Geometry check sheet. Reference: drawing and pictorial views, mm from the part's lowest x, y, z. A direction names the side the tool comes from. Round coordinates to 2 decimals unless told otherwise and drop trailing zeros. Order: outer loops, then holes, each group sorted by start corner. A loop starts at its lowest first (then second) coordinate and runs counter-clockwise, first axis right, second up. Notation, with made-up numbers: (8.5, 60.25) -> (22.5, 60.25) arc R31 cw to (22.5, 91.25) -> close; hole circle Ø5 at (-31.75, 65). An arc over 180 degrees is marked (long way). Put each result on its own line as item: value.
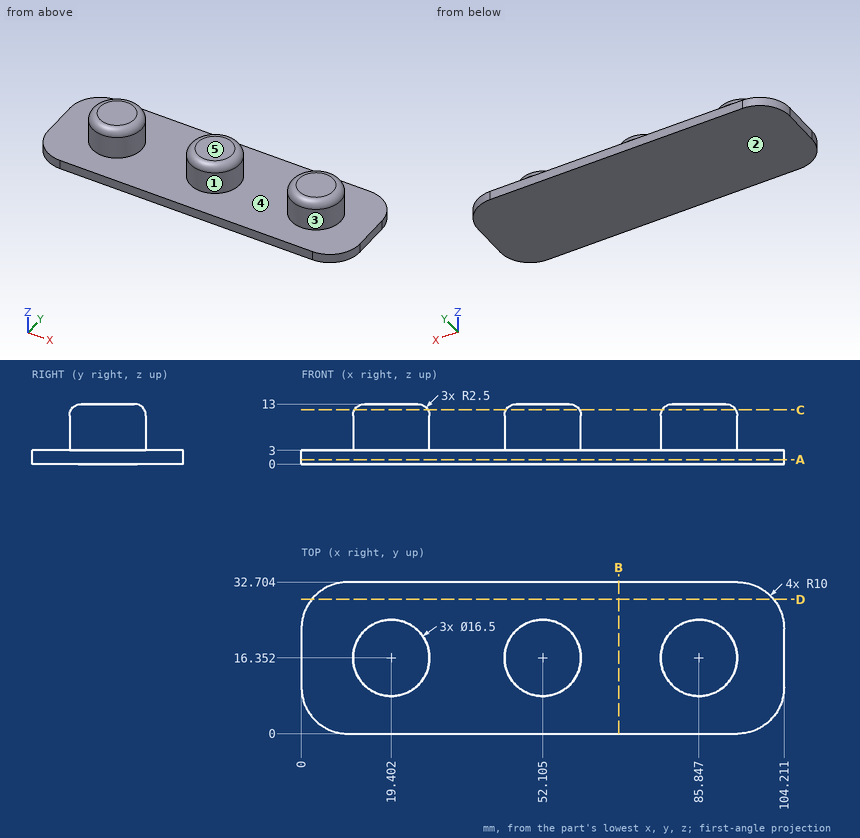
Item 1: Tool access check on the marked faces 1 and 2. Record the directions out of +Z, -Z, +X, -X, +Y, -Y that give a thin tool (end or side, any length) a straight path to the whole face; none if there is none.
Geometry check:
face 1: +Z
face 2: -Z, +X, -X, +Y, -Y
Item 2: Sectioned sample at B-B, the plane x = 68.5. Record the boundary of the cut face in (y, z).
Geometry check:
outline: (0, 0) -> (32.7, 0) -> (32.7, 3) -> (0, 3) -> close
Item 3: Material ranges on line 1 along X through (y, z) = (11.5, 8) (1 decimal); line 2 along X through (y, z) = (12, 7.25) (1 decimal); line 3 along Z through (x, y) = (92, 26), recorded low to high.
Geometry check:
line 1: 12.7 to 26.1, 45.4 to 58.8, 79.2 to 92.5
line 2: 12.4 to 26.4, 45.1 to 59.1, 78.8 to 92.9
line 3: 0 to 3
Item 4: Sectioned sample at D-D, the plane y = 29. Record the boundary of the cut face in (x, z), then the cut area to 3 significant figures.
Geometry check:
outline: (2.23, 0) -> (101.98, 0) -> (101.98, 3) -> (2.23, 3) -> close
area: 299 mm2
Item 5: Release check for a two-part mould opening along X. For the marked faces 3, 4 and 5 record: pulls with the +X half, pulls with the -X half, needs draft (parallel to the pull), parting line crosses it, or undercut.
Geometry check:
face 3: undercut
face 4: undercut
face 5: needs draft
Item 6: Sectioned sample at A-A, the plane z = 1. Record the boundary of the cut face in (x, y), then the cut area to 3 significant figures.
Geometry check:
outline: (0, 10) arc R10 ccw to (10, 0) -> (94.21, 0) arc R10 ccw to (104.21, 10) -> (104.21, 22.7) arc R10 ccw to (94.21, 32.7) -> (10, 32.7) arc R10 ccw to (0, 22.7) -> close
area: 3,320 mm2
Item 7: Depth check by flat-ended pin: pin 1 Ø2 at (x, y) = (94, 19) entering from +Z; pin 2 Ø2 at (x, z) = (82.5, 5.5) entering from +Y; pin 3 Ø6 at (y, z) = (7.5, 9) entering from -X (1 decimal). Enter the tip coordinate at first touch or a pass-through.
Geometry check:
pin 1: z = 12.21
pin 2: y = 24.26
pin 3: x = 13.6
Item 8: Sectioned sample at C-C, the plane z = 11.75. Record the boundary of the cut face in (x, y) (1 decimal).
Geometry check:
outline: circle Ø15.8 at (19.4, 16.4); circle Ø15.8 at (52.1, 16.4); circle Ø15.8 at (85.8, 16.4)
